```python
from build123d import *

# Parameters (mm, degrees)
SKETCH1_W          = 40
SKETCH1_H          = 40
SKETCH3_R          = 5
CUT_EXTRUDE1_DEPTH = 70.282032476


with BuildPart() as part:
    # Sketch1 → Loft1 section 0
    with BuildSketch(Plane(origin=(0, 0, 0), x_dir=(1, 0, 0), z_dir=(0, 1, 0))):
        with Locations((20, 20)):
            Rectangle(SKETCH1_W, SKETCH1_H)
    # Sketch2 for Loft1 → Loft1 section 1
    with BuildSketch(Plane(origin=(0, 40, 0), x_dir=(1, 0, 0), z_dir=(0, 1, 0))):
        with BuildLine():
            # circular arc as an exact rational Bezier (weights 1, cos(half-angle), 1)
            Bezier((12.928932188, 12.928932188), (20, 5.857864377), (27.071067812, 12.928932188), weights=[1, 0.707106781, 1])
            Bezier((27.071067812, 12.928932188), (34.142135623, 20), (27.071067812, 27.071067812), weights=[1, 0.707106781, 1])
            Bezier((27.071067812, 27.071067812), (20, 34.142135623), (12.928932188, 27.071067812), weights=[1, 0.707106781, 1])
            Bezier((12.928932188, 27.071067812), (5.857864377, 20), (12.928932188, 12.928932188), weights=[1, 0.707106781, 1])
        make_face()
    loft()

    # Sketch3 → Cut-Extrude1 (cut, through all)
    with BuildSketch(Plane(origin=(0, 40, 0), x_dir=(1, 0, 0), z_dir=(0, 1, 0))):
        with Locations(Location((20, 20, 0), (0, 0, 270))):
            Circle(SKETCH3_R)
    extrude(amount=-CUT_EXTRUDE1_DEPTH, mode=Mode.SUBTRACT)


solid = part.part
```
The listing builds one solid part. Answer for the finished solid, in the listing's coordinates (mm). Give positions to 0.01 mm unless a question says otherwise; leave off trailing zeros. Return JSON: item names as keys, results as strings. Group by question number.
1. Determine the mould class of faces 1 (the cylindrical face through (15.12, 20.28, -21.08)), 2 (the flat face through (15, 0, -24)) for opening direction X: pulls with the +X half, pulls with the -X half, needs draft (parallel to the pull), parting line crosses it, or undercut.
2. Straight lines are drawn through the part: line 1 (X direction, y = 28, z = -20); line 2 (X direction, y = 23.5, z = -18.5); line 3 (Z direction, x = 18, y = 24). For each, find the intervals that lie inside material, in ascending order. Write a range as [from, to].
3. Given pin 1 Ø10 at (x, y) = (23, 15.5) entering from +Z; pin 2 Ø10 at (y, z) = (17, -17.5) entering from -X; pin 3 Ø8 at (x, y) = (7, 15) entering from -Z, each flat-ended and moving along its own axis, determine where each tip first touches the part or whether it passes through.
Verdict:
{
 "1": {"face 1": "undercut", "face 2": "needs draft"},
 "2": {"line 1": "x = [7, 15], [25, 33]", "line 2": "x = [5.9, 15.23], [24.77, 34.1]", "line 3": "z = [-33.95, -24.58], [-15.42, -6.05]"},
 "3": {"pin 1": "stops at z = -2.65", "pin 2": "stops at x = 3.02", "pin 3": "stops at z = -36.76"}
}
